Here's how the part is built. I have some questions about the finished solid (model axes, mm). A direction names the side the tool comes from. Coordinates: 2 decimals unless noted, no trailing zeros. Write each loop counter-clockwise with the first axis right and the second up, starting at its lowest first coordinate (ties: lowest second). Pieces come first, ordered by that corner, then holes. Notation, with made-up numbers: (13.25, 88) -> (23.25, 88) arc R14 ccw to (23.25, 92) -> close; hole circle Ø11 at (-21.75, 24.5). An arc over 180 degrees is marked (long way). Put each result on its own line as item: value.
```python
from build123d import *

# Parameters (mm, degrees)
F0_R     = 9
F1_DEPTH = 50


with BuildPart() as f1:
    # F0 (on Top) → F1 (new body)
    with BuildSketch(Plane.XY):
        with BuildLine():
            ThreePointArc((49.38715, -7.804448), (49.846552, -3.914237), (50, 0))
            ThreePointArc((50, 0), (49.846552, 3.914237), (49.38715, 7.804448))
            ThreePointArc((49.38715, 7.804448), (35.355339, 35.355339), (7.804448, 49.38715))
            ThreePointArc((7.804448, 49.38715), (0, 50), (-7.804448, 49.38715))
            ThreePointArc((-7.804448, 49.38715), (-35.355339, 35.355339), (-49.38715, 7.804448))
            ThreePointArc((-49.38715, 7.804448), (-50, 0), (-49.38715, -7.804448))
            ThreePointArc((-49.38715, -7.804448), (-35.355339, -35.355339), (-7.804448, -49.38715))
            ThreePointArc((-7.804448, -49.38715), (0, -50), (7.804448, -49.38715))
            ThreePointArc((7.804448, -49.38715), (35.355339, -35.355339), (49.38715, -7.804448))
        make_face()
        Circle(F0_R, mode=Mode.SUBTRACT)
        with BuildLine():
            ThreePointArc((-7.804448, 49.38715), (0, 50), (7.804448, 49.38715))
            Line((7.804448, 49.38715), (7.804448, 58.050208))
            Line((7.804448, 58.050208), (-7.804448, 58.050208))
            Line((-7.804448, 58.050208), (-7.804448, 49.38715))
        make_face()
        with BuildLine():
            ThreePointArc((49.38715, 7.804448), (49.846552, 3.914237), (50, 0))
            ThreePointArc((50, 0), (49.846552, -3.914237), (49.38715, -7.804448))
            Line((49.38715, -7.804448), (58.050208, -7.804448))
            Line((58.050208, -7.804448), (58.050208, 7.804448))
            Line((58.050208, 7.804448), (49.38715, 7.804448))
        make_face()
        with BuildLine():
            Line((7.804448, -58.050208), (7.804448, -49.38715))
            ThreePointArc((7.804448, -49.38715), (0, -50), (-7.804448, -49.38715))
            Line((-7.804448, -49.38715), (-7.804448, -58.050208))
            Line((-7.804448, -58.050208), (7.804448, -58.050208))
        make_face()
        with BuildLine():
            ThreePointArc((-49.38715, -7.804448), (-50, 0), (-49.38715, 7.804448))
            Line((-49.38715, 7.804448), (-58.050208, 7.804448))
            Line((-58.050208, 7.804448), (-58.050208, -7.804448))
            Line((-58.050208, -7.804448), (-49.38715, -7.804448))
        make_face()
    extrude(amount=F1_DEPTH)


solid = f1.part
```
Item 1: Imagine slicing it at D-D on x = 51. Write out the boundary of the cut face in (y, z), then the cut area to 3 significant figures.
Output:
outline: (-7.8, 0) -> (7.8, 0) -> (7.8, 50) -> (-7.8, 50) -> close
area: 780 mm²
Item 2: Imagine slicing it at C-C on z = 5. Write out the boundary of the cut face in (x, y), then the cut area to 3 significant figures.
Output:
outline: (-58.05, -7.8) -> (-49.39, -7.8) arc R50 ccw to (-7.8, -49.39) -> (-7.8, -58.05) -> (7.8, -58.05) -> (7.8, -49.39) arc R50 ccw to (49.39, -7.8) -> (58.05, -7.8) -> (58.05, 7.8) -> (49.39, 7.8) arc R50 ccw to (7.8, 49.39) -> (7.8, 58.05) -> (-7.8, 58.05) -> (-7.8, 49.39) arc R50 ccw to (-49.39, 7.8) -> (-58.05, 7.8) -> close; hole circle Ø18 at (0, 0)
area: 8,110 mm²
Item 3: If we mould it in two halves opening along Y, with no side actions, what happens to faces 1 (the flat face through (54, 7.804, 25)), 2 (the flat face through (12, 1, 0)), 3 (the cylindrical face through (-1.172, 8.923, 24.65))? For each: released by +Y, released by -Y, zero draft, split by the parting line, or undercut.
Output:
face 1: released by +Y
face 2: zero draft
face 3: undercut
Item 4: Which directions (+Z, -Z, +X, -X, +Y, -Y) give clear straight access to the entire face, cutting with the end or side of a thin tool? Please do faces 4 (the flat face through (-7.804, -54, 25)), 5 (the flat face through (7.804, -54, 25)), 6 (the flat face through (7.804, 54, 25)), 7 (the flat face through (-7.804, 54, 25)), 8 (the flat face through (0, 58.05, 25)).
Output:
face 4: +Z, -Z, -X, -Y
face 5: +Z, -Z, +X, -Y
face 6: +Z, -Z, +X, +Y
face 7: +Z, -Z, -X, +Y
face 8: +Z, -Z, +X, -X, +Y
Item 5: Please list where these lines run through material, in increasing order: line 1 along Y through (x, z) = (0, 33); line 2 along X through (y, z) = (52, 46.5); line 3 along X through (y, z) = (-5.5, 10.5). Write a range as from..to.
Output:
line 1: y = -58.05..-9, 9..58.05
line 2: x = -7.8..7.8
line 3: x = -58.05..-7.12, 7.12..58.05
Item 6: For P1, Ø6, axis at x = 41, z = 44, coming from the +Y side; P2, Ø7, axis at x = 53, z = 23.5, coming from the -Y side; P3, Ø9.5, axis at x = 54.5, z = 22.5, coming from the +Y side; P4, Ø10, axis at x = -10.5, z = 40, coming from the +Y side, each with a flat end and sliding along its axis, tell me the tip position at first contact or that it passes through.
Output:
P1: stops at y = 32.5
P2: stops at y = -7.8
P3: stops at y = 7.8
P4: stops at y = 58.05
Item 7: Imagine slicing it at A-A on y = 0. Write out the boundary of the cut face in (x, z).
Output:
outline: (-58.05, 0) -> (-9, 0) -> (-9, 50) -> (-58.05, 50) -> close; (9, 0) -> (58.05, 0) -> (58.05, 50) -> (9, 50) -> close
